CAD build for the part. Positions are in the model's coordinates, mm. Coordinates: 2 decimals unless noted, no trailing zeros. Order: outer loops, then holes, each group sorted by start corner. A loop starts at its lowest first (then second) coordinate and runs counter-clockwise, first axis right, second up. Notation, with made-up numbers: (-35, -10.5) -> (-6, -10.5) arc R20 cw to (-6, 13.5) -> close; hole circle Ø9 at (-8.5, 34.25). An arc over 180 degrees is marked (long way). Use one line per item in the form item = value. Start each with the question number.
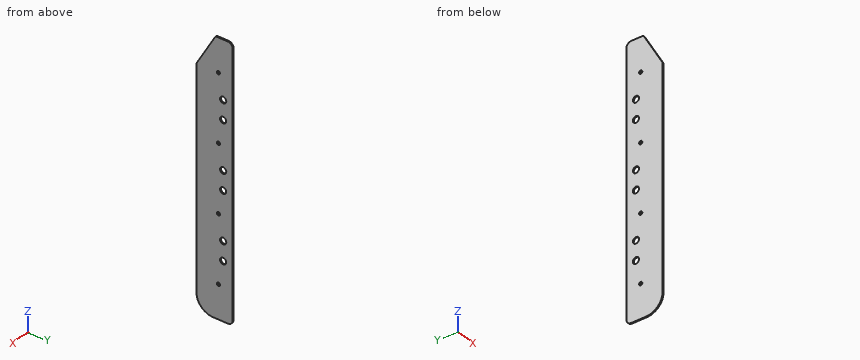
Autodesk Inventor part; units mm, degrees
ref_plane "YZ Plane" through (0, 0, 0) normal (1, 0, 0) x (0, 1, 0)
ref_plane "XZ Plane" through (0, 0, 0) normal (0, 1, 0) x (-1, 0, 0)
ref_plane "XY Plane" through (0, 0, 0) normal (0, 0, 1) x (1, 0, 0)
sketch "main" plane through (0, 0, 0) normal (0, 0, 1) x (1, 0, 0)
  circle A0 centre (-6.8277, 139.0371) radius 2.1844
  circle A1 centre (-0.4777, 107.2871) radius 4.191
  line L0 (-8.7029, 183.4871) -> (6.7737, 183.4871)
  circle A2 centre (-6.8277, 50.1371) radius 2.1844
  circle A3 centre (-6.8277, -38.7629) radius 2.1844
  circle A4 centre (-6.8277, -127.6629) radius 2.1844
  circle A5 centre (-0.4777, 81.8871) radius 4.191
  circle A6 centre (-0.4777, 18.3871) radius 4.191
  line L1 (-36.1964, -149.8879) -> (-36.1964, 139.0371)
  circle A7 centre (-0.4777, -70.5129) radius 4.191
  circle A8 centre (-0.4777, -95.9129) radius 4.191
  line L2 (6.7053, -172.1129) -> (5.8723, -172.1129)
  line L3 (-13.9714, -172.1129) -> (6.7053, -172.1129)
  arc A9 (-36.1964, -149.8879) -> (-13.9714, -172.1129) centre (-13.9714, -149.8879) ccw
  circle A10 centre (-0.4777, -7.0129) radius 4.191
  line L4 (-11.4526, 181.8995) -> (-36.1964, 139.0371)
  arc A11 (-8.7029, 183.4871) -> (-11.4526, 181.8995) centre (-8.7029, 180.3121) ccw
  line L5 (-8.7029, 183.4871) -> (5.8723, 183.4871)
  line L6 (12.2223, 177.1371) -> (12.2223, -165.7629)
  arc A12 (12.2223, 177.1371) -> (5.8723, 183.4871) centre (5.8723, 177.1371) ccw
  arc A13 (5.8723, -172.1129) -> (12.2223, -165.7629) centre (5.8723, -165.7629) ccw
  point P0 (2.0753, 1.669)
  point P1 (-10.536, 183.4871)
  point P2 (5.8723, 139.0371)
  point P3 (12.2223, 183.4871)
  dimension "d4" = 8.382
  dimension "d5" = 8.382
  dimension "d6" = 8.382
  dimension "d7" = 8.382
  dimension "d8" = 8.382
  dimension "d9" = 8.382
  dimension "d10" = 12.7
  dimension "d11" = 0
  dimension "d12" = 88.9
  dimension "d13" = 88.9
  dimension "d14" = 88.9
  dimension "d15" = 29.3687
  dimension "d16" = 3.175
  dimension "d18" = 6.35
  dimension "d19" = 6.35
  dimension "d20" = 22.225
sketch "Sketch1" plane through (0, 0, 0) normal (1, 0, 0) x (0, 1, 0)
  circle A0 centre (0, 0) radius 2.1844
  circle A1 centre (6.35, -31.75) radius 4.191
  line L0 (-1.8752, 44.45) -> (13.6014, 44.45)
  circle A2 centre (0, -88.9) radius 2.1844
  circle A3 centre (0, -177.8) radius 2.1844
  circle A4 centre (0, -266.7) radius 2.1844
  circle A5 centre (6.35, -57.15) radius 4.191
  circle A6 centre (6.35, -120.65) radius 4.191
  line L1 (-29.3687, -288.925) -> (-29.3687, 0)
  circle A7 centre (6.35, -209.55) radius 4.191
  circle A8 centre (6.35, -234.95) radius 4.191
  line L2 (13.533, -311.15) -> (12.7, -311.15)
  line L3 (-7.1437, -311.15) -> (13.533, -311.15)
  arc A9 (-29.3687, -288.925) -> (-7.1437, -311.15) centre (-7.1437, -288.925) ccw
  circle A10 centre (6.35, -146.05) radius 4.191
  line L4 (-4.6249, 42.8624) -> (-29.3687, 0)
  arc A11 (-1.8752, 44.45) -> (-4.6249, 42.8624) centre (-1.8752, 41.275) ccw
  line L5 (-1.8752, 44.45) -> (12.7, 44.45)
  line L6 (19.05, 38.1) -> (19.05, -304.8)
  arc A12 (19.05, 38.1) -> (12.7, 44.45) centre (12.7, 38.1) ccw
  arc A13 (12.7, -311.15) -> (19.05, -304.8) centre (12.7, -304.8) ccw
extrude "Extrusion1" add sketch "Sketch1" along normal blind 1.5875
properties part number "Skirt" material "Acetal Resin, White"
1) Drop a flat-ended pin along its axis: P1, Ø5.5, axis at y = 0, z = -266.7, coming from the -X side. Give the stop position or say it passes through.
2) Cut at C-C on x = 1. Count the separate pieces of the cut face and the enclosed holes in it, then the cut area to 3 significant figures.
3) Cut at A-A on y = 6.35. Give the cut face in (x, z), then the cut area to 3 significant figures.
4) Cut at B-B on z = -234.95. Give the cut face in (x, y), then the cut area to 3 significant figures.
5) Cut at D-D on y = -12. Give the cut face in (x, z), then the cut area to 3 significant figures.
6) Probe L1, parallel to Z at x = 0.45, y = 0; L2, parallel to Y at x = 0.4, z = -177.5; L3, parallel to Y at x = 1.25, z = -118. List the from-to ranges inside material, lowest first.
Values follow:
q1.P1 = 0
q2.separate_pieces = 1
q2.enclosed_holes = 10
q2.area = 16,100 mm^2
q3.outline = (0, -311.15) -> (1.59, -311.15) -> (1.59, -239.14) -> (0, -239.14) -> close; (0, -230.76) -> (1.59, -230.76) -> (1.59, -213.74) -> (0, -213.74) -> close; (0, -205.36) -> (1.59, -205.36) -> (1.59, -150.24) -> (0, -150.24) -> close; (0, -141.86) -> (1.59, -141.86) -> (1.59, -124.84) -> (0, -124.84) -> close; (0, -116.46) -> (1.59, -116.46) -> (1.59, -61.34) -> (0, -61.34) -> close; (0, -52.96) -> (1.59, -52.96) -> (1.59, -35.94) -> (0, -35.94) -> close; (0, -27.56) -> (1.59, -27.56) -> (1.59, 44.45) -> (0, 44.45) -> close
q3.area = 485 mm^2
q4.outline = (0, -29.37) -> (1.59, -29.37) -> (1.59, 2.16) -> (0, 2.16) -> close; (0, 10.54) -> (1.59, 10.54) -> (1.59, 19.05) -> (0, 19.05) -> close
q4.area = 63.6 mm^2
q5.outline = (0, -310.61) -> (1.59, -310.61) -> (1.59, 30.09) -> (0, 30.09) -> close
q5.area = 541 mm^2
q6.L1 = -311.15 to -268.88, -264.52 to -179.98, -175.62 to -91.08, -86.72 to -2.18, 2.18 to 44.45
q6.L2 = -29.37 to -2.16, 2.16 to 19.05
q6.L3 = -29.37 to 3.1, 9.6 to 19.05
